Autodesk Inventor part; units mm, degrees
ref_plane "YZ Plane" through (0, 0, 0) normal (1, 0, 0) x (0, 1, 0)
ref_plane "XZ Plane" through (0, 0, 0) normal (0, 1, 0) x (-1, 0, 0)
ref_plane "XY Plane" through (0, 0, 0) normal (0, 0, 1) x (1, 0, 0)
sketch "Esboço1" plane through (0, 0, 0) normal (0, 1, 0) x (-1, 0, 0)
  line L0 (0, 5) -> (-5, 5)
  line L1 (60, -55) -> (60, -60)
  line L2 (60, -60) -> (-5, -60)
  line L3 (-5, -60) -> (-5, 5)
  line L4 (-5, 5) -> (60, 5)
  line L5 (60, 5) -> (60, -60)
  line L6 (27.5, 5) -> (32.5, 5)
  circle A0 centre (32.5, -27.5) radius 7.25
  dimension "d11" = 5
  dimension "d13" = 5
  dimension "d16" = 5
  dimension "d17" = 14.5
extrude "Extrusão4" add sketch "Esboço1" along normal blind 1
sketch "Esboço2" plane through (0, 1, 0) normal (0, 1, 0) x (1, 0, 0)
  circle A0 centre (-32.5, 27.5) radius 7.25
  circle A1 centre (-4.5, 27.5) radius 1.5
  point P0 (0, 0)
  dimension "d21" = 3
extrude "Extrusão5" cut sketch "Esboço2" against normal blind 10 contours A1
pattern_circular "Padrão circular1" count 3 over 360 about axis through (-32.5, 0, -27.5) along (0, 1, 0) of "Extrusão5"
sketch "Esboço3" plane through (-60, 0, 5) normal (0, 0, 1) x (1, 0, 0)
  line L0 (65, 0) -> (0, 0)
  line L1 (65, 1) -> (0, 1)
  line L2 (0, 1) -> (0, 0)
  line L3 (0, 0) -> (65, 0)
  line L4 (65, 0) -> (65, 1)
  point P0 (60, 0)
sketch "Esboço4" plane through (5, 0, -60) normal (0, 0, -1) x (-1, 0, 0)
  line L0 (0, 1) -> (65, 1)
  line L1 (65, 1) -> (0, 1)
  line L2 (0, 1) -> (0, 0)
  line L3 (0, 0) -> (65, 0)
  line L4 (65, 0) -> (65, 1)
  point P0 (5, 0)
fillet "Arredondamento1" radius 3 4 edges at (5, 0.5, -60) (5, 0.5, 5) (-60, 0.5, -60) (-60, 0.5, 5)
properties part number "borracha isolamento respirador" material "Borracha"
The model under review builds one solid part; all positions refer to its coordinate system, in mm. Round coordinates to 2 decimals unless told otherwise and drop trailing zeros. Write each loop counter-clockwise with the first axis right and the second up, starting at its lowest first coordinate (ties: lowest second). Pieces come first, ordered by that corner, then holes. Notation, with made-up numbers: M 50,-31 L 80,-31 A24 ccw 80,-18 Z; hole C 55.25,69.25 d8. An arc over 180 degrees is marked long. Use a Markdown table: item, result. Add a question column.
Q1. We need section C-C, the plane x = -46.5. State the section outline as (y, z) points.
Q2. We need section B-B, the plane x = -32.5. State the section outline as (y, z) points, plus the area to 3 significant figures.
Q3. We need section A-A, the plane z = -27.5. State the section outline as (x, y) points, plus the area to 3 significant figures.
Q4. We need section D-D, the plane y = 0.85. State the section outline as (x, z) points.
Q5. To check wall thickness, follow line 1 (X direction, y = 0.35, z = -27); line 2 (Z direction, x = -32.5, y = 0.6); line 3 (Z direction, x = -4.5, y = 0.85). State the ranges of each line that lie inside material, in increasing order.
Q6. The part is to be moulded in two halves that separate along X. For faces 1 (the face through (4.1, 0.51, 4.14)), 2 (the face through (-59.14, 0.51, 4.1)), 3 (the face through (-47.61, 0.51, -52.76)), say which applies: pulls with the +X half, pulls with the -X half, needs draft (parallel to the pull), parting line crosses it, or undercut.
Findings below:
| question | item | result |
|---|---|---|
| 1 | outline | M 0,-60 L 1,-60 L 1,-53.25 L 0,-53.25 Z; M 0,-50.25 L 1,-50.25 L 1,-4.75 L 0,-4.75 Z; M 0,-1.75 L 1,-1.75 L 1,5 L 0,5 Z |
| 2 | outline | M 0,-60 L 1,-60 L 1,-34.75 L 0,-34.75 Z; M 0,-20.25 L 1,-20.25 L 1,5 L 0,5 Z |
| 2 | area | 50.5 mm² |
| 3 | outline | M -60,0 L -39.75,0 L -39.75,1 L -60,1 Z; M -25.25,0 L -6,0 L -6,1 L -25.25,1 Z; M -3,0 L 5,0 L 5,1 L -3,1 Z |
| 3 | area | 47.5 mm² |
| 4 | outline | M -60,-57 A3 ccw -57,-60 L 2,-60 A3 ccw 5,-57 L 5,2 A3 ccw 2,5 L -57,5 A3 ccw -60,2 Z; hole C -46.5,-51.75 d3; hole C -46.5,-3.25 d3; hole C -32.5,-27.5 d14.5; hole C -4.5,-27.5 d3 |
| 5 | line 1 | x = -60 to -39.73, -25.27 to -5.91, -3.09 to 5 |
| 5 | line 2 | z = -60 to -34.75, -20.25 to 5 |
| 5 | line 3 | z = -60 to -29, -26 to 5 |
| 6 | face 1 | pulls with the +X half |
| 6 | face 2 | pulls with the -X half |
| 6 | face 3 | undercut |
